Here's how the part is built. I have some questions about the finished solid (model axes, mm). Face numbers are marked on the shaded views. A direction names the side the tool comes from. Coordinates: 2 decimals unless noted, no trailing zeros. Order: outer loops, then holes, each group sorted by start corner. A loop starts at its lowest first (then second) coordinate and runs counter-clockwise, first axis right, second up. Notation, with made-up numbers: (31.25, -13.75) - (89.25, -13.75) arc R19 ccw to (89.25, 5.25) - close; hole circle Ø5 at (52, 59). An arc over 180 degrees is marked (long way). Answer in a Markdown table with one row per item. Add a question column.
Item 1: I want a section at D-D (y = 12). Please give me the cut outline in (x, z), plus the area to 3 significant figures.
Item 2: Will these pins go through, and if not, where does the flat tip stop? pin 1 Ø12 at (x, y) = (-0.5, 31.5) entering from +Z; pin 2 Ø3 at (x, y) = (6.5, 47) entering from -Z; pin 3 Ø2.5 at (y, z) = (73.5, -7) entering from -X.
Item 3: I want a section at C-C (y = 71). Please give me the cut outline in (x, z).
Item 4: I want a section at B-B (x = 0). Please give me the cut outline in (y, z).
Item 5: I want a section at A-A (z = 0). Please give me the cut outline in (x, y).
Item 6: If I drill on line 1 along X through (y, z) = (63, -0.5); line 2 along X through (y, z) = (58.5, -0.5); line 3 along Y through (x, z) = (2, 9.5), over which ranges is the centre line in solid material (lowest first)? Write a range as from..to.
Item 7: On a 3-axis mill with a long thin cutter (end or side, diameter ignored), from which of +Z, -Z, +X, -X, +Y, -Y can I reach the whole of each face in a straight line? I mean the marked faces 1, 2 and 3. Say none if no direction works.
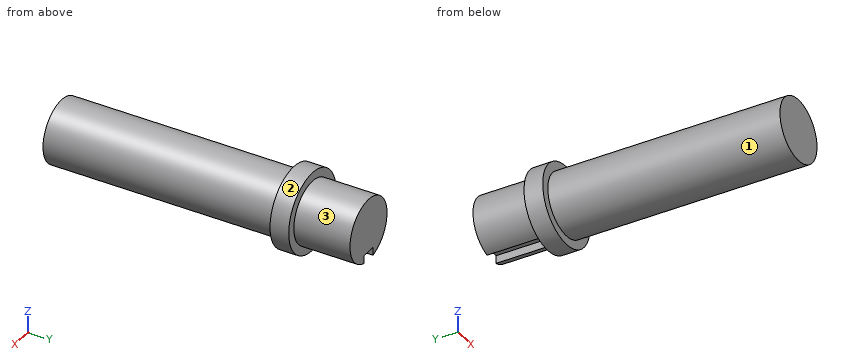
```python
from build123d import *

# Parameters (mm, degrees)
SKETCH1_R           = 8.35
BOSS_EXTRUDE1_DEPTH = 82
SKETCH2_R           = 10.65
BOSS_EXTRUDE2_DEPTH = 5
SKETCH3_W           = 4
SKETCH3_H           = 8.442622751
CUT_EXTRUDE1_DEPTH  = 15


with BuildPart() as part:
    # Sketch1 → Boss-Extrude1 (new body)
    with BuildSketch(Plane(origin=(0, 0, 0), x_dir=(1, 0, 0), z_dir=(0, 1, 0))):
        with Locations(Location((0, 0, 0), (0, 0, 270))):
            Circle(SKETCH1_R)
    extrude(amount=BOSS_EXTRUDE1_DEPTH)

    # Sketch2 → Boss-Extrude2 (add)
    with BuildSketch(Plane(origin=(0, 62, 0), x_dir=(1, 0, 0), z_dir=(0, 1, 0))):
        with Locations(Location((0, 0, 0), (0, 0, 270))):
            Circle(SKETCH2_R)
    extrude(amount=BOSS_EXTRUDE2_DEPTH)

    # Sketch3 → Cut-Extrude1 (cut)
    with BuildSketch(Plane(origin=(0, 82, 0), x_dir=(1, 0, 0), z_dir=(0, 1, 0))):
        with Locations((0, 10.221311376)):
            Rectangle(SKETCH3_W, SKETCH3_H)
    extrude(amount=-CUT_EXTRUDE1_DEPTH, mode=Mode.SUBTRACT)


solid = part.part
```
Values follow:
| question | item | result |
|---|---|---|
| 1 | outline | circle Ø16.7 at (0, 0) |
| 1 | area | 219 mm^2 |
| 2 | pin 1 | stops at z = 8.35 |
| 2 | pin 2 | stops at z = -6.69 |
| 2 | pin 3 | stops at x = -6.05 |
| 3 | outline | (-2, -8.11) - (-2, -6) - (2, -6) - (2, -8.11) arc R8.35 ccw (long way) to start |
| 4 | outline | (0, -8.35) - (62, -8.35) - (62, -10.65) - (67, -10.65) - (67, -6) - (82, -6) - (82, 8.35) - (67, 8.35) - (67, 10.65) - (62, 10.65) - (62, 8.35) - (0, 8.35) - close |
| 5 | outline | (-10.65, 62) - (-8.35, 62) - (-8.35, 0) - (8.35, 0) - (8.35, 62) - (10.65, 62) - (10.65, 67) - (8.35, 67) - (8.35, 82) - (-8.35, 82) - (-8.35, 67) - (-10.65, 67) - close |
| 6 | line 1 | x = -10.64..10.64 |
| 6 | line 2 | x = -8.34..8.34 |
| 6 | line 3 | y = 62..67 |
| 7 | face 1 | -Y |
| 7 | face 2 | +Y, -Y |
| 7 | face 3 | +Y |
